Design review of the part built by this model. Coordinates are the model's own, in mm. A direction names the side the tool comes from. Round coordinates to 2 decimals unless told otherwise and drop trailing zeros. Loops run counter-clockwise (first coordinate to the right, second up) from the corner with the lowest first, then second, coordinate; pieces in that order, holes last. Notation, with made-up numbers: (-15, -9.75) - (-3, -9.75) arc R28 ccw to (-3, 13.25) - close; hole circle Ø10 at (-32.75, 81). An arc over 180 degrees is marked (long way). Return JSON: item names as keys, results as strings. Group by question number.
(1) Wall thickness on L1, parallel to Z at x = -40, y = 1.35; L2, parallel to Z at x = 39, y = -0.5; L3, parallel to Y at x = -20.5, z = 36.5: over which ranges is each line inside the solid? List them lowest first. Write a range as [from, to].
(2) For faces 5 (the cylindrical face through (53.3, -1.2, -49.4)), 6 (the cylindrical face through (-34.2, -1.2, -49.4)), 7 (the cylindrical face through (-53.6, -1.2, 49.2)), list the 3-axis set-ups (+Z, -Z, +X, -X, +Y, -Y) from which the entire face can be reached by the end or side of a thin tool; tool diameter is ignored.
(3) We need section B-B, the plane z = 17.5. Write out the cut boundary in (x, y), and give its area (3 significant figures).
(4) The part is to be moulded in two halves that separate along X. For faces 1 (the flat face through (59.75, 17, -1)), 2 (the flat face through (-59.75, 17, 1)), 3 (the cylindrical face through (-34.2, -1.2, 49.4)), 4 (the cylindrical face through (33.15, -1.23, 49.21)), say which applies: pulls with the +X half, pulls with the -X half, needs draft (parallel to the pull), parting line crosses it, or undercut.
(5) Clearance check with flat-ended pins moving along their axes: pin 1 (0.8 mm diameter, centred on x = 43.5, y = -1, fed in from +Z); pin 2 (2 mm diameter, centred on x = 40, z = 0.5, fed in from -Y); pin 3 (0.8 mm diameter, centred on x = -41.5, y = -1.5, fed in from -Z). State where each tip first meets the part, or that it passes through.
(6) We need section A-A, the plane x = -4. Write out the cut boundary in (y, z), and give its area (3 significant figures).
Autodesk Fusion 360 part; units mm, degrees
sketch "Sketch1" plane through (0, 0, 0) normal (0, 1, 0) x (1, 0, 0)
  line L0 (59.75, -59.75) -> (-59.75, -59.75)
  line L1 (-59.75, -59.75) -> (-59.75, 59.75)
  line L2 (-59.75, 59.75) -> (59.75, 59.75)
  line L3 (59.75, 59.75) -> (59.75, -59.75)
  line L4 (59.75, -59.75) -> (-59.75, 59.75) construction
  line L5 (-59.75, -59.75) -> (59.75, 59.75) construction
  dimension "d2" = 119.5
extrude "Extrude1" add sketch "Sketch1" along normal blind 34.7
fillet "Fillet1" radius 10 4 edges at (-59.75, 17.35, 59.75) (59.75, 17.35, 59.75) (-59.75, 17.35, -59.75) (59.75, 17.35, -59.75)
sketch "Sketch4" plane through (0, 0, 0) normal (0, -1, 0) x (1, 0, 0)
  line L0 (-49.75, -59.75) -> (49.75, -59.75)
  line L1 (59.75, -49.75) -> (59.75, 49.75)
  line L2 (49.75, 59.75) -> (-49.75, 59.75)
  line L3 (-59.75, 49.75) -> (-59.75, -49.75)
  line L4 (-49.4, 45.1) -> (-38.4, 45.1)
  arc A0 (-38.4, 45.1) -> (-38.4, 53.5) centre (-38.4, 49.3) ccw
  line L5 (-38.4, 53.5) -> (-49.4, 53.5)
  arc A1 (-49.4, 53.5) -> (-49.4, 45.1) centre (-49.4, 49.3) ccw
  line L6 (-49.4, 49.3) -> (-38.4, 49.3) construction
  line L7 (-49.4, -53.7) -> (-38.4, -53.7)
  arc A2 (-38.4, -53.7) -> (-38.4, -45.3) centre (-38.4, -49.5) ccw
  line L8 (-38.4, -45.3) -> (-49.4, -45.3)
  arc A3 (-49.4, -45.3) -> (-49.4, -53.7) centre (-49.4, -49.5) ccw
  line L9 (-49.4, -49.5) -> (-38.4, -49.5) construction
  line L10 (49.1, -45.3) -> (38.1, -45.3)
  arc A4 (38.1, -45.3) -> (38.1, -53.7) centre (38.1, -49.5) ccw
  line L11 (38.1, -53.7) -> (49.1, -53.7)
  arc A5 (49.1, -53.7) -> (49.1, -45.3) centre (49.1, -49.5) ccw
  line L12 (49.1, -49.5) -> (38.1, -49.5) construction
  line L13 (37.35, 45.1) -> (48.35, 45.1)
  arc A6 (48.35, 45.1) -> (48.35, 53.5) centre (48.35, 49.3) ccw
  line L14 (48.35, 53.5) -> (37.35, 53.5)
  arc A7 (37.35, 53.5) -> (37.35, 45.1) centre (37.35, 49.3) ccw
  line L15 (37.35, 49.3) -> (48.35, 49.3) construction
  arc A8 (49.75, -59.75) -> (59.75, -49.75) centre (49.75, -49.75) ccw
  arc A9 (59.75, 49.75) -> (49.75, 59.75) centre (49.75, 49.75) ccw
  arc A10 (-49.75, 59.75) -> (-59.75, 49.75) centre (-49.75, 49.75) ccw
  arc A11 (-59.75, -49.75) -> (-49.75, -59.75) centre (-49.75, -49.75) ccw
  dimension "d6" = 4.2
  dimension "d7" = 11
  dimension "d8" = 49.4
  dimension "d9" = 49.3
  dimension "d14" = 37.35
  dimension "d15" = 49.5
  dimension "d16" = 49.1
extrude "Extrude2" add sketch "Sketch4" along normal blind 2.5 contours L4 A0 L5 A1 | L7 A2 L8 A3 | L10 A4 L11 A5 | L13 A6 L14 A7
sketch "Sketch5" plane through (0, 0, 0) normal (0, -1, 0) x (1, 0, 0)
  line L0 (37.35, 53.5) -> (48.35, 53.5)
  arc A0 (48.35, 45.1) -> (48.35, 53.5) centre (48.35, 49.3) ccw
  line L1 (48.35, 45.1) -> (37.35, 45.1)
  arc A1 (37.35, 53.5) -> (37.35, 45.1) centre (37.35, 49.3) ccw
  line L2 (-49.4, 53.5) -> (-38.4, 53.5)
  arc A2 (-38.4, 45.1) -> (-38.4, 53.5) centre (-38.4, 49.3) ccw
  line L3 (-38.4, 45.1) -> (-49.4, 45.1)
  arc A3 (-49.4, 53.5) -> (-49.4, 45.1) centre (-49.4, 49.3) ccw
  line L4 (49.1, -53.7) -> (38.1, -53.7)
  arc A4 (38.1, -45.3) -> (38.1, -53.7) centre (38.1, -49.5) ccw
  line L5 (38.1, -45.3) -> (49.1, -45.3)
  arc A5 (49.1, -53.7) -> (49.1, -45.3) centre (49.1, -49.5) ccw
  line L6 (-49.4, -45.3) -> (-38.4, -45.3)
  arc A6 (-38.4, -53.7) -> (-38.4, -45.3) centre (-38.4, -49.5) ccw
  line L7 (-38.4, -53.7) -> (-49.4, -53.7)
  arc A7 (-49.4, -45.3) -> (-49.4, -53.7) centre (-49.4, -49.5) ccw
  line L8 (-49.75, -59.75) -> (49.75, -59.75)
  line L9 (59.75, -49.75) -> (59.75, 49.75)
  line L10 (49.75, 59.75) -> (-49.75, 59.75)
  line L11 (-59.75, 49.75) -> (-59.75, -49.75)
  line L12 (-40, 0) -> (40, 0) construction
  circle A8 centre (-40, 0) radius 1.25
  circle A9 centre (40, 0) radius 1.25
  arc A10 (49.75, -59.75) -> (59.75, -49.75) centre (49.75, -49.75) ccw
  arc A11 (59.75, 49.75) -> (49.75, 59.75) centre (49.75, 49.75) ccw
  arc A12 (-49.75, 59.75) -> (-59.75, 49.75) centre (-49.75, 49.75) ccw
  arc A13 (-59.75, -49.75) -> (-49.75, -59.75) centre (-49.75, -49.75) ccw
  dimension "d17" = 2.5
  dimension "d18" = 80
extrude "Extrude3" cut sketch "Sketch5" against normal blind 3 contours A8 | A9
Solutions:
{
 "1": {"L1": "[-59.75, -1.25], [1.25, 59.75]", "L2": "[-53.7, -45.3], [45.1, 53.5]", "L3": "[0, 34.7]"},
 "2": {"face 5": "+X, -Y", "face 6": "-Y", "face 7": "-X, -Y"},
 "3": {"outline": "(-59.75, 0) - (59.75, 0) - (59.75, 34.7) - (-59.75, 34.7) - close", "area": "4,150 mm^2"},
 "4": {"face 1": "pulls with the +X half", "face 2": "pulls with the -X half", "face 3": "undercut", "face 4": "undercut"},
 "5": {"pin 1": "z = 53.5", "pin 2": "y = 0", "pin 3": "z = -53.7"},
 "6": {"outline": "(0, -59.75) - (34.7, -59.75) - (34.7, 59.75) - (0, 59.75) - close", "area": "4,150 mm^2"}
}
